from build123d import *

# Parameters (mm, degrees)
BOSS_EXTRUDE1_DEPTH      = 30
BOSS_EXTRUDE1_DEPTH_BACK = 30
SKETCH2_W                = 600
SKETCH2_H                = 800
SKETCH2_W_2              = 500
SKETCH2_H_2              = 700
SKETCH3_R                = 25
BOSS_EXTRUDE2_DEPTH      = 62.5


with BuildPart() as part:
    # Sketch2 → Boss-Extrude1 (new, two sides: drawn at the far end of the back side and taken through both)
    with BuildSketch(Plane.XY.offset(-BOSS_EXTRUDE1_DEPTH_BACK)):
        Rectangle(SKETCH2_W, SKETCH2_H)
        Rectangle(SKETCH2_W_2, SKETCH2_H_2, mode=Mode.SUBTRACT)
    extrude(amount=BOSS_EXTRUDE1_DEPTH + BOSS_EXTRUDE1_DEPTH_BACK)

    # Sketch3 → Boss-Extrude2 (add)
    with BuildSketch(Plane(origin=(300, 0, 0), x_dir=(0, 0, -1), z_dir=(1, 0, 0))):
        with Locations(Location((0, 0, 0), (0, 0, 90))):
            Circle(SKETCH3_R)
    boss_extrude2 = extrude(amount=BOSS_EXTRUDE2_DEPTH)

    # Mirror1: Boss-Extrude2 across plane
    add(boss_extrude2.mirror(Plane(origin=(0, 0, 0), x_dir=(0, 0, 1), z_dir=(1, 0, 0))))


solid = part.part
Work out the finished part from the listing and answer in its coordinate system (mm). A direction names the side the tool comes from. Coordinates: 2 decimals unless noted, no trailing zeros. Loops run counter-clockwise (first coordinate to the right, second up) from the corner with the lowest first, then second, coordinate; pieces in that order, holes last. Notation, with made-up numbers: M 85.5,22.5 L 119.5,22.5 A26 ccw 119.5,56.5 Z; hole C -12,38 d5. An arc over 180 degrees is marked long. Answer in a Markdown table with one row per item. Add a question column.
1. Find section A-A, the plane x = 133.5. Write down the section's boundary in (y, z).
2. A flat-ended cylindrical pin translates along its axis: P1, Ø3, axis at y = -211, z = 21, coming from the +X side. Find the tip coordinate at first contact, or state that the pin passes through.
3. Find section D-D, the plane y = 150. Write down the section's boundary in (x, z).
4. Consider L1, parallel to Y at x = -84, z = 13; L2, parallel to X at y = -186.5, z = -20; L3, parallel to Y at x = -327, z = -5. Determine where each line is inside the solid, lowest interval first.
5. A tool of negligible diameter and unlimited length cuts with its end or side. For faces 4 (the cylindrical face through (330.812, 23.846, 7.509)), 5 (the flat face through (-268, 2, -30)), 6 (the cylindrical face through (-330.812, 23.846, 7.509)), 7 (the flat face through (-3, -350, 0)), 8 (the flat face through (362.5, 0, 0)), from which of +Z, -Z, +X, -X, +Y, -Y can it reach the whole face along a straight path? Write none if from no direction.
6. Find section B-B, the plane y = 0. Write down the section's boundary in (x, z), then the cut area to 4 significant figures.
7. The mould has two halves that part along X. Classify faces 1 (the flat face through (-362.5, 0, 0)), 2 (the flat face through (-4, -400, 0)), 3 (the flat face through (-250, -5, 0)): pulls with the +X half, pulls with the -X half, needs draft (parallel to the pull), parting line crosses it, or undercut.
8. Find section C-C, the plane z = 0. Write down the section's boundary in (x, y), then the cut area to 3 significant figures.
Reported:
| question | item | result |
|---|---|---|
| 1 | outline | M -400,-30 L -350,-30 L -350,30 L -400,30 Z; M 350,-30 L 400,-30 L 400,30 L 350,30 Z |
| 2 | P1 | stops at x = 300 |
| 3 | outline | M -300,-30 L -250,-30 L -250,30 L -300,30 Z; M 250,-30 L 300,-30 L 300,30 L 250,30 Z |
| 4 | L1 | y = -400 to -350, 350 to 400 |
| 4 | L2 | x = -300 to -250, 250 to 300 |
| 4 | L3 | y = -24.49 to 24.49 |
| 5 | face 4 | +X |
| 5 | face 5 | -Z, +X, -X, +Y, -Y |
| 5 | face 6 | -X |
| 5 | face 7 | +Z, -Z |
| 5 | face 8 | +Z, -Z, +X, +Y, -Y |
| 6 | outline | M -362.5,-25 L -300,-25 L -300,-30 L -250,-30 L -250,30 L -300,30 L -300,25 L -362.5,25 Z; M 250,-30 L 300,-30 L 300,-25 L 362.5,-25 L 362.5,25 L 300,25 L 300,30 L 250,30 Z |
| 6 | area | 12,250 mm^2 |
| 7 | face 1 | pulls with the -X half |
| 7 | face 2 | needs draft |
| 7 | face 3 | undercut |
| 8 | outline | M -362.5,-25 L -300,-25 L -300,-400 L 300,-400 L 300,-25 L 362.5,-25 L 362.5,25 L 300,25 L 300,400 L -300,400 L -300,25 L -362.5,25 Z; hole M -250,-350 L 250,-350 L 250,350 L -250,350 Z |
| 8 | area | 136,000 mm^2 |
